Design review of the part built by this model. Coordinates are the model's own, in mm. A direction names the side the tool comes from. Round coordinates to 2 decimals unless told otherwise and drop trailing zeros. Write each loop counter-clockwise with the first axis right and the second up, starting at its lowest first coordinate (ties: lowest second). Pieces come first, ordered by that corner, then holes. Notation, with made-up numbers: M -14.75,12 L 10.25,12 A11 ccw 10.25,32 Z; hole C -24,63 d3. An arc over 180 degrees is marked long. One line per question, with ' | ' between items. Start each with the question number.
Item 1: Add section B-B, the plane x = -13.5. State the section outline as (y, z) points.
Item 2: Insertion check: pin 1 Ø1.5 at (x, y) = (9, 1) entering from -Z. The pin has a flat end and moves straight along its axis. Give the tip position at first contact, or say it passes through.
Item 3: Add section A-A, the plane z = -0.75. State the section outline as (x, y) points, and give its area (3 significant figures).
Item 4: Machinability: for faces 1 (the face through (0, 7.5, 0)), 2 (the face through (18.732, 5.599, -1.325)), which of the approach directions +Z, -Z, +X, -X, +Y, -Y give a long, thin tool a straight path to every point of the face, cutting with its end or side? Answer none if there is none.
Item 5: For L1, parallel to X at y = 3.25, z = 4; L2, parallel to Z at x = -1, y = 0.75; L3, parallel to Z at x = -4.5, y = 5.75, list the stretches that pass through material, from the lowest coordinate up.
Item 6: Add section C-C, the plane z = -4.25. State the section outline as (x, y) points, and give its area (3 significant figures).
Item 7: Draft analysis for pull direction Z (two halves, no side actions). For faces 3 (the face through (-17.5, 4, 0)), 4 (the face through (0, 4, -8.5)), 5 (the face through (18.732, 5.866, 0.593)), 6 (the face through (0.25, 6.9, 7.93)), state which applies: released by +Z, released by -Z, zero draft, split by the parting line, or undercut.
```python
from build123d import *

# Parameters (mm, degrees)
SKETCH1_W           = 35
SKETCH1_H           = 17
BOSS_EXTRUDE1_DEPTH = 7.5
CHAMFER1_SIZE       = 2
CHAMFER1_SIZE2      = 2.856296013
FILLET1_R           = 2
SKETCH3_R           = 0.725
BOSS_EXTRUDE2_DEPTH = 2.5


with BuildPart() as part:
    # Sketch1 → Boss-Extrude1 (new body)
    with BuildSketch(Plane(origin=(0, 0, 0), x_dir=(1, 0, 0), z_dir=(0, 1, 0))):
        Rectangle(SKETCH1_W, SKETCH1_H)
    extrude(amount=BOSS_EXTRUDE1_DEPTH)

    # Chamfer1
    chamfer1_edges = [part.edges().sort_by_distance(p)[0] for p in [
        (17.5, 0, 0),
    ]]
    chamfer1_side = [part.faces().sort_by_distance(p)[0] for p in [
        (0, 0, 0),
    ]]
    chamfer(chamfer1_edges, length=CHAMFER1_SIZE, length2=CHAMFER1_SIZE2, reference=chamfer1_side[0])

    # Fillet1
    fillet1_edges = [part.edges().sort_by_distance(p)[0] for p in [
        (-1, 0, -8.5),
        (0, 7.5, 8.5),
        (-1, 0, 8.5),
        (0, 7.5, -8.5),
    ]]
    fillet(fillet1_edges, radius=FILLET1_R)

    # Sketch3 → Boss-Extrude2 (add)
    with BuildSketch(Plane(origin=(17.5, 0, 0), x_dir=(0, 0, -1), z_dir=(1, 0, 0))):
        with Locations(Location((-0.75, 5.157979839, 0), (0, 0, 180))):
            Circle(SKETCH3_R)
        with Locations(Location((0.75, 5.157979839, 0), (0, 0, 180))):
            Circle(SKETCH3_R)
    extrude(amount=BOSS_EXTRUDE2_DEPTH)


solid = part.part
```
Computed values:
1) outline: M 0,-6.5 A2 ccw 2,-8.5 L 5.5,-8.5 A2 ccw 7.5,-6.5 L 7.5,6.5 A2 ccw 5.5,8.5 L 2,8.5 A2 ccw 0,6.5 Z
2) pin 1: stops at z = -8.48
3) outline: M -17.5,0 L 15.5,0 L 17.5,2.86 L 17.5,4.43 L 20,4.43 L 20,5.88 L 17.5,5.88 L 17.5,7.5 L -17.5,7.5 Z | area: 263 mm^2
4) face 1: +Z, -Z, +X, -X, +Y | face 2: +X
5) L1: x = -17.5 to 17.5 | L2: z = -8.06 to 8.06 | L3: z = -8.48 to 8.48
6) outline: M -17.5,0 L 15.5,0 L 17.5,2.86 L 17.5,7.5 L -17.5,7.5 Z | area: 260 mm^2
7) face 3: zero draft | face 4: released by -Z | face 5: undercut | face 6: released by +Z
